Source: three-view drawing plus pictorial views. Frame: mm from the lowest corner of the part. Give positions to 0.01 mm unless a question says otherwise; leave off trailing zeros. Loops run counter-clockwise (first coordinate to the right, second up) from the corner with the lowest first, then second, coordinate; pieces in that order, holes last. Notation, with made-up numbers: (27, 80) -> (67, 80) arc R15 cw to (67, 90) -> close; hole circle Ø9 at (29.25, -28). An arc over 180 degrees is marked (long way). Put each result on its own line as item: value.
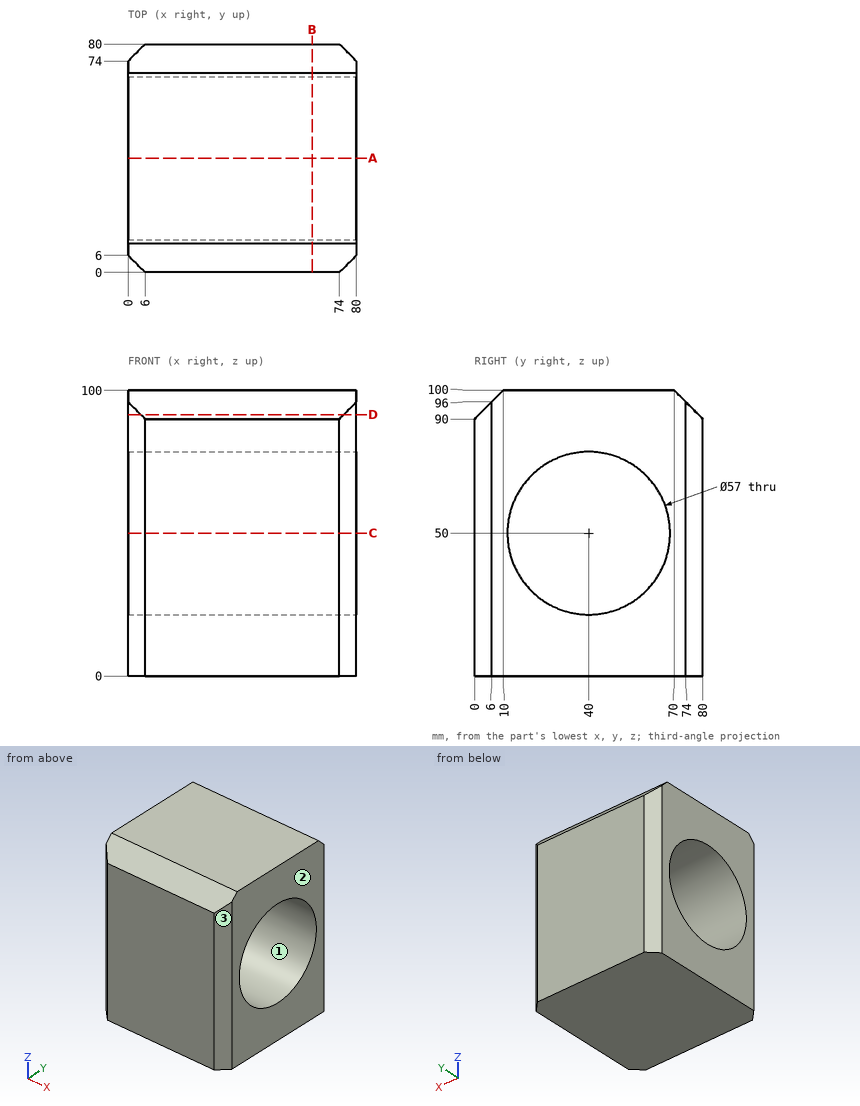
(1) First-contact query: P1, Ø10, axis at x = 20, y = 71, coming from the +Z side. Flat tip, straight axial feed; report the tip coordinate or a pass-through.
Calculated:
P1: stops at z = 100
(2) Section D-D on z = 91.5. Return loops of the section in (x, y), then the cut area to 3 significant figures.
Calculated:
outline: (0, 6) -> (4.5, 1.5) -> (75.5, 1.5) -> (80, 6) -> (80, 74) -> (75.5, 78.5) -> (4.5, 78.5) -> (0, 74) -> close
area: 6,120 mm²
(3) Line query: probe 1 along Y at (x, z) = (32, 50); probe 2 along Z at (x, y) = (5, 19); probe 3 along Y at (x, z) = (62.5, 62). Output: solid intervals per line, ascending. Write a range as from..to.
Calculated:
probe 1: y = 0..11.5, 68.5..80
probe 2: z = 0..30.73, 69.27..100
probe 3: y = 0..14.15, 65.85..80
(4) Section C-C on z = 50. Return loops of the section in (x, y), then the cut area to 3 significant figures.
Calculated:
outline: (0, 6) -> (6, 0) -> (74, 0) -> (80, 6) -> (80, 11.5) -> (0, 11.5) -> close; (0, 68.5) -> (80, 68.5) -> (80, 74) -> (74, 80) -> (6, 80) -> (0, 74) -> close
area: 1,770 mm²
(5) Section A-A on y = 40. Return loops of the section in (x, z), then the cut area to 3 significant figures.
Calculated:
outline: (0, 0) -> (80, 0) -> (80, 21.5) -> (0, 21.5) -> close; (0, 78.5) -> (80, 78.5) -> (80, 100) -> (0, 100) -> close
area: 3,440 mm²
(6) Section B-B on x = 64.5. Return loops of the section in (y, z).
Calculated:
outline: (0, 0) -> (80, 0) -> (80, 90) -> (70, 100) -> (10, 100) -> (0, 90) -> close; hole circle Ø57 at (40, 50)
(7) Draft query along Y for the marked faces 1, 2 and 3. Return one class per face: released by +Y, released by -Y, zero draft, split by the parting line, or undercut.
Calculated:
face 1: undercut
face 2: zero draft
face 3: released by -Y
